Build history of the part. All positions in model axes, mm. Face numbers are marked on the shaded views. A direction names the side the tool comes from. Coordinates: 2 decimals unless noted, no trailing zeros. Loops run counter-clockwise (first coordinate to the right, second up) from the corner with the lowest first, then second, coordinate; pieces in that order, holes last.
(1) Slice it at A-A (y = -92.5). Give the cut face in (x, z), and give its area (3 significant figures).
(2) Flat gauge pins, fed straight in: P1, Ø4, axis at x = 50, y = 50, coming from the -Z side; P2, Ø4.5, axis at x = -50, y = -50, coming from the +Z side; P3, Ø4.5, axis at x = -50, y = 50, coming from the -Z side. Where does each tip first touch, or does it go through?
(3) Slice it at B-B (x = 1.5). Give the cut face in (y, z).
(4) Tool access for the marked faces 1 and 2: list every direction of +Z, -Z, +X, -X, +Y, -Y with a clear straight run to the whole face (end or side of a thin tool).
(5) Wall check: L1, parallel to Y at x = 50, z = 11; L2, parallel to X at y = 50, z = 7; L3, parallel to Z at x = 217.5, y = 1.5. Give the ranges that are in metal, low to high.
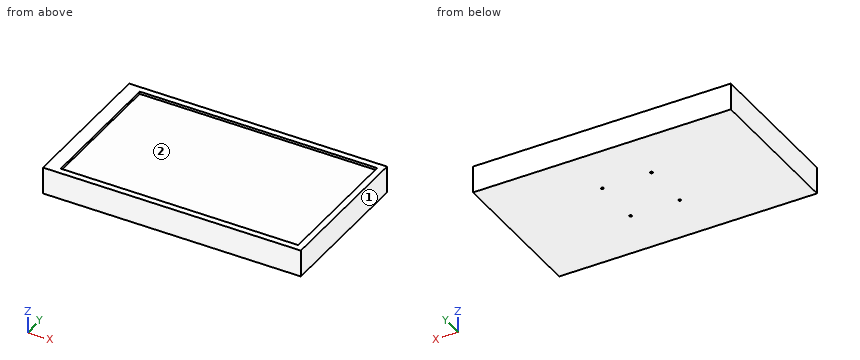
from build123d import *

# Parameters (mm, degrees)
SKETCH2_W                 = 508
SKETCH2_H                 = 304.8
BOSS_EXTRUDE1_DEPTH       = 55
M6X1_0_TAPPED_HOLE1_D     = 5
M6X1_0_TAPPED_HOLE1_DEPTH = 17
M6X1_0_TAPPED_HOLE1_TIP   = 1.502151548
SKETCH6_W                 = 482.6
SKETCH6_H                 = 279.4
CUT_EXTRUDE1_DEPTH        = 5
SKETCH7_W                 = 55
SKETCH7_H                 = 304.8
BOSS_EXTRUDE2_DEPTH       = 16


with BuildPart() as part:
    # Sketch2 → Boss-Extrude1 (new body)
    with BuildSketch(Plane.XY):
        Rectangle(SKETCH2_W, SKETCH2_H)
    extrude(amount=BOSS_EXTRUDE1_DEPTH)

    # M6x1.0 Tapped Hole1
    with Locations(Plane(origin=(0, 0, 0), x_dir=(-1, 0, 0), z_dir=(0, 0, -1))):
        with Locations((50, 50), (-50, -50), (-50, 50), (50, -50)):
            Hole(M6X1_0_TAPPED_HOLE1_D / 2, depth=M6X1_0_TAPPED_HOLE1_DEPTH)
            with Locations((0, 0, -(M6X1_0_TAPPED_HOLE1_DEPTH + M6X1_0_TAPPED_HOLE1_TIP / 2))):  # 118° drill point
                Cone(0, M6X1_0_TAPPED_HOLE1_D / 2, M6X1_0_TAPPED_HOLE1_TIP, mode=Mode.SUBTRACT)

    # Sketch6 → Cut-Extrude1 (cut)
    with BuildSketch(Plane.XY.offset(55)):
        Rectangle(SKETCH6_W, SKETCH6_H)
    extrude(amount=-CUT_EXTRUDE1_DEPTH, mode=Mode.SUBTRACT)

    # Sketch7 → Boss-Extrude2 (add)
    with BuildSketch(Plane.ZY.offset(254)):
        with Locations((27.5, 0)):
            Rectangle(SKETCH7_W, SKETCH7_H)
    extrude(amount=BOSS_EXTRUDE2_DEPTH)


solid = part.part
Response values:
1. outline: (-270, 0) - (254, 0) - (254, 55) - (241.3, 55) - (241.3, 50) - (-241.3, 50) - (-241.3, 55) - (-270, 55) - close
1. area: 26,400 mm2
2. P1: stops at z = 17.3
2. P2: stops at z = 50
2. P3: stops at z = 17.15
3. outline: (-152.4, 0) - (152.4, 0) - (152.4, 55) - (139.7, 55) - (139.7, 50) - (-139.7, 50) - (-139.7, 55) - (-152.4, 55) - close
4. face 1: +Z, -Z, +X, +Y, -Y
4. face 2: +Z
5. L1: y = -152.4 to -52.5, -47.5 to 47.5, 52.5 to 152.4
5. L2: x = -270 to -52.5, -47.5 to 47.5, 52.5 to 254
5. L3: z = 0 to 50
